from build123d import *

# Parameters (mm, degrees)
SKETCH_1_W          = 46
SKETCH_1_H          = 32
EXTRUDE_1_DEPTH     = 18
SKETCH_2_W          = 63
SKETCH_2_H          = 1.528020249
EXTRUDE_2_DEPTH     = 32
CUT_EXTRUDE_1_DEPTH = 39.981740814
FILLET_1_R          = 0.558031
FILLET_2_R          = 0.558031
FILLET_3_R          = 0.558031
FILLET_4_R          = 0.558031
SKETCH_5_R          = 1.5
EXTRUDE_3_DEPTH     = 10


with BuildPart() as part:
    # 草图1 → 凸台-拉伸1 (new body)
    with BuildSketch(Plane(origin=(0, 0, 0), x_dir=(1, 0, 0), z_dir=(0, 1, 0))):
        Rectangle(SKETCH_1_W, SKETCH_1_H)
    extrude(amount=EXTRUDE_1_DEPTH)

    # 草图2 → 凸台-拉伸2 (add, through all)
    with BuildSketch(Plane.XY.offset(16)):
        with Locations((0, 0.764010125)):
            Rectangle(SKETCH_2_W, SKETCH_2_H)
    extrude(amount=-EXTRUDE_2_DEPTH)

    # 草图3 → 切除-拉伸1 (cut, through all)
    with BuildSketch(Plane(origin=(0, 1.528020249, 0), x_dir=(1, 0, 0), z_dir=(0, 1, 0))):
        Polygon((-31.5, 16), (-31.5, 3), (-23, 5), (-23, 16), align=None)
        Polygon((-23, -5), (-31.5, -3), (-31.5, -16), (-23, -16), align=None)
        with BuildLine():
            ThreePointArc((-28, -2), (-26, 0), (-28, 2))
            Line((-28, 2), (-31.5, 2))
            Line((-31.5, 2), (-31.5, -2))
            Line((-31.5, -2), (-28, -2))
        make_face()
    cut_extrude_1 = extrude(amount=-CUT_EXTRUDE_1_DEPTH, mode=Mode.SUBTRACT)

    # 圆角1
    fillet_1_edges = [part.edges().sort_by_distance(p)[0] for p in [
        (-31.5, 0.764010125, -3),
        (-31.5, 0.764010125, -2),
    ]]
    fillet(fillet_1_edges, radius=FILLET_1_R)

    # 圆角2
    fillet_2_edges = [part.edges().sort_by_distance(p)[0] for p in [
        (-31.5, 0.764010125, 3),
        (-31.5, 0.764010125, 2),
    ]]
    fillet(fillet_2_edges, radius=FILLET_2_R)

    # 镜向4: 切除-拉伸1 across plane
    add(cut_extrude_1.mirror(Plane(origin=(0, 0, 0), x_dir=(0, 0, 1), z_dir=(1, 0, 0))), mode=Mode.SUBTRACT)

    # 圆角3
    fillet_3_edges = [part.edges().sort_by_distance(p)[0] for p in [
        (31.5, 0.764010125, -3),
        (31.5, 0.764010125, -2),
    ]]
    fillet(fillet_3_edges, radius=FILLET_3_R)

    # 圆角4
    fillet_4_edges = [part.edges().sort_by_distance(p)[0] for p in [
        (31.5, 0.764010125, 3),
        (31.5, 0.764010125, 2),
    ]]
    fillet(fillet_4_edges, radius=FILLET_4_R)

    # 草图5 → 凸台-拉伸3 (add)
    with BuildSketch(Plane.XY.offset(16)):
        with Locations(Location((-16.963649323, 4.593857319, 0), (0, 0, 180))):
            Circle(SKETCH_5_R)
        with Locations(Location((-11.147540984, 4.593857319, 0), (0, 0, 180))):
            Circle(SKETCH_5_R)
        with Locations(Location((11.147540984, 4.593857319, 0), (0, 0, 180))):
            Circle(SKETCH_5_R)
        with Locations(Location((16.963649323, 4.593857319, 0), (0, 0, 180))):
            Circle(SKETCH_5_R)
    extrude(amount=EXTRUDE_3_DEPTH)


solid = part.part
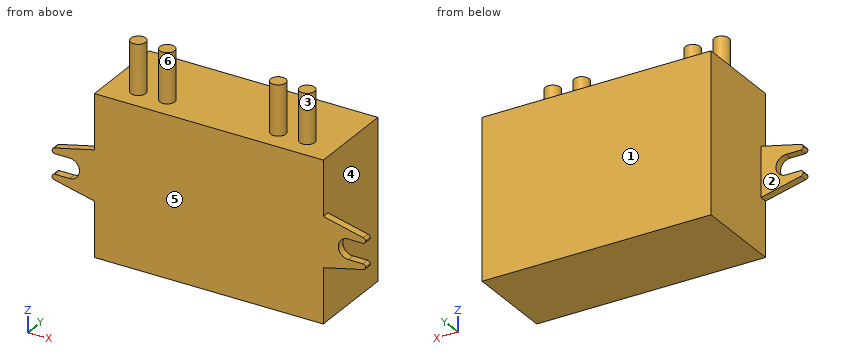
Geometry check sheet. Reference: the model listing, model coordinates, mm. Face numbers are marked on the shaded views. A direction names the side the tool comes from. Round coordinates to 2 decimals unless told otherwise and drop trailing zeros. Loops run counter-clockwise (first coordinate to the right, second up) from the corner with the lowest first, then second, coordinate; pieces in that order, holes last. Notation, with made-up numbers: (83, 14) -> (133, 14) arc R21 cw to (133, 45) -> close; hole circle Ø1 at (89.25, -28). An arc over 180 degrees is marked (long way). Answer as a JSON object with one key per item and string values. Group by question number.
Item 1: Set-up check for the marked faces 1, 2 and 3: record each of +Z, -Z, +X, -X, +Y, -Y from which the full face is reachable in a straight line by a thin tool's end or side.
Item 2: Cross-section at A-A, the plane z = 0. Record the cut outline in (x, y).
Item 3: Release check for a two-part mould opening along X. For the marked faces 4, 5 and 6 record: pulls with the +X half, pulls with the -X half, needs draft (parallel to the pull), parting line crosses it, or undercut.
Item 4: Depth check by flat-ended pin: pin 1 Ø1.2 at (x, y) = (-30, 0.5) entering from -Z; pin 2 Ø10 at (y, z) = (2, -1) entering from -X; pin 3 Ø1.7 at (x, y) = (-29.5, 1) entering from +Z; pin 4 Ø4 at (y, z) = (10, 17.5) entering from +X. Enter the tip coordinate at first touch or a pass-through.
Item 5: Cross-section at C-C, the plane y = 13. Record the cut outline in (x, z).
Item 6: Cross-section at B-B, the plane x = -13.5. Record the cut outline in (y, z).
Item 7: Thickness scan on line 1 along Z through (x, y) = (1, 8.75); line 2 along X through (y, z) = (1, 6); line 3 along Y through (x, z) = (-24, 4). Record the ranges inside material, lowest first.
Determined:
{
 "1": {"face 1": "+Z, -Z, +X, -X, +Y", "face 2": "+Z, -Z, -X, +Y", "face 3": "+Z"},
 "2": {"outline": "(-26, 0) -> (26, 0) -> (26, 1.53) -> (23, 1.53) -> (23, 18) -> (-23, 18) -> (-23, 1.53) -> (-26, 1.53) -> close"},
 "3": {"face 4": "pulls with the +X half", "face 5": "needs draft", "face 6": "undercut"},
 "4": {"pin 1": "stops at z = -3.49", "pin 2": "stops at x = -31.5", "pin 3": "stops at z = 3.67", "pin 4": "stops at x = 23"},
 "5": {"outline": "(-23, -16) -> (23, -16) -> (23, 16) -> (-23, 16) -> close"},
 "6": {"outline": "(0, -16) -> (18, -16) -> (18, 16) -> (0, 16) -> close"},
 "7": {"line 1": "z = -16 to 16", "line 2": "x = -23 to 23", "line 3": "y = 0 to 1.53"}
}
